Geometry: final body of the model. Coordinates: model frame, mm. Face numbers are marked on the shaded views. A direction names the side the tool comes from. Give positions to 0.01 mm unless a question says otherwise; leave off trailing zeros. Write each loop counter-clockwise with the first axis right and the second up, starting at its lowest first coordinate (ties: lowest second). Pieces come first, ordered by that corner, then holes. Notation, with made-up numbers: (75.5, 84) -> (91.5, 84) arc R27 ccw to (91.5, 106) -> close; hole circle Ø10 at (13, 81.5). An arc over 180 degrees is marked (long way). Answer as a JSON object with one key per item and string values.
from build123d import *

# Parameters (mm, degrees)
BOSS_EXTRUDE1_DEPTH = 308
SKETCH2_R           = 3
CUT_EXTRUDE1_DEPTH  = 310.295974756


with BuildPart() as part:
    # Sketch1 → Boss-Extrude1 (new body)
    with BuildSketch(Plane(origin=(0, 0, 0), x_dir=(0, 0, -1), z_dir=(1, 0, 0))):
        Polygon((0, 0), (20, 0), (20, 3.461178467), (3.461178467, 3.461178467), (3.461178467, 20), (0, 20), align=None)
    extrude(amount=BOSS_EXTRUDE1_DEPTH)

    # Sketch2 → Cut-Extrude1 (cut, through all)
    with BuildSketch(Plane.XY):
        with Locations((278, 11.75)):
            Circle(SKETCH2_R)
        Polygon((308, 10), (298, 20), (308, 20), align=None)
    extrude(amount=-CUT_EXTRUDE1_DEPTH, mode=Mode.SUBTRACT)


solid = part.part
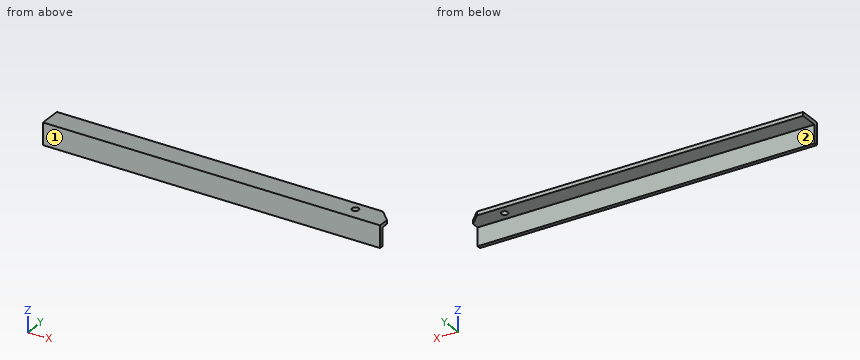
Q1. Cut plane C-C (z = -12). Return the cut outline in (x, y), and give its area (3 significant figures).
Values:
{"outline": "(0, 0) -> (308, 0) -> (308, 3.46) -> (0, 3.46) -> close", "area": "1,070 mm²"}
Q2. Set-up query: the marked faces 1 and 2. Return all of +Z, -Z, +X, -X, +Y, -Y with unobstructed straight access to the full face (end or side cutting, diameter ignored); none if empty.
Values:
{"face 1": "+Z, -Z, +X, -X, -Y", "face 2": "-Z, +X, -X, +Y"}
Q3. First-contact query: P1, Ø5, axis at x = 190, y = 13, coming from the -Z side; P2, Ø3, axis at y = 3, z = -11, coming from the -X side; P3, Ø5.5, axis at x = 278, y = 11.75, coming from the +Z side. Flat tips, straight axial feed; report the tip coordinate or a pass-through.
Values:
{"P1": "z = -3.46", "P2": "x = 0", "P3": "through"}
Q4. Cut plane B-B (x = 233). Return the cut outline in (y, z).
Values:
{"outline": "(0, -20) -> (3.46, -20) -> (3.46, -3.46) -> (20, -3.46) -> (20, 0) -> (0, 0) -> close"}
Q5. Cut plane A-A (x = 278). Return the cut outline in (y, z), and give its area (3 significant figures).
Values:
{"outline": "(0, -20) -> (3.46, -20) -> (3.46, -3.46) -> (8.75, -3.46) -> (8.75, 0) -> (0, 0) -> close; (14.75, -3.46) -> (20, -3.46) -> (20, 0) -> (14.75, 0) -> close", "area": "106 mm²"}
Q6. Material intervals for L1, parallel to Y at x = 278, z = -2.05; L2, parallel to Z at x = 70, y = 8.5; L3, parallel to Y at x = 153.5, z = -9, sorted ascending. Write a range as from..to.
Values:
{"L1": "0..8.75, 14.75..20", "L2": "-3.46..0", "L3": "0..3.46"}
